```python
from build123d import *

# Parameters (mm, degrees)
F0_W     = 40
F0_H     = 20
F1_DEPTH = 700
F2_SIZE2 = 3.52653
F2_SIZE  = 19.99999
F3_SIZE2 = 3.52653
F3_SIZE  = 19.99999


# Not quite as in the source:
# - a fillet or chamfer is up to 0.001 mm smaller than in the source, because OpenCascade refuses the exact size


with BuildPart() as f1:
    # F0 (on Front) → F1 (new body)
    with BuildSketch(Plane.XZ):
        with Locations((20, 10)):
            Rectangle(F0_W, F0_H)
    extrude(amount=F1_DEPTH)

    # F2 (size 20 and 3.5265396142 in the source; OpenCascade refuses exactly that, so slightly less here)
    f2_edges = [f1.edges().sort_by_distance(p)[0] for p in [
        (20, -700, 0),
    ]]
    f2_side = f1.faces().sort_by_distance((20, -700, 10))[0]
    chamfer(f2_edges, length=F2_SIZE, length2=F2_SIZE2, reference=f2_side)

    # F3 (size 20 and 3.5265396142 in the source; OpenCascade refuses exactly that, so slightly less here)
    f3_edges = [f1.edges().sort_by_distance(p)[0] for p in [
        (20, 0, 0),
    ]]
    f3_side = f1.faces().sort_by_distance((20, 0, 10))[0]
    chamfer(f3_edges, length=F3_SIZE, length2=F3_SIZE2, reference=f3_side)


solid = f1.part
```
Here's how the part is built. I have some questions about the finished solid (model axes, mm). Give positions to 0.01 mm unless a question says otherwise; leave off trailing zeros. Use a Markdown table: item, result. Add a question column.
1. For pin 1 Ø5 at (x, z) = (5, 9.5) entering from -Y; pin 2 Ø6 at (x, z) = (12.5, 3.5) entering from -Y; pin 3 Ø6 at (y, z) = (-169, 17) entering from -X; pin 4 Ø5 at (x, z) = (31, 15) entering from +Y, each with a flat end and sliding along its axis, tell me the tip position at first contact or that it passes through.
2. I need wall thicknesses on probe 1 along Y at (x, z) = (29.5, 10.75); probe 2 along Y at (x, z) = (4.5, 1.5). Which ranges of each line are inside material? Lowest first, please. Write a range as from..to.
3. If we mould it in two halves opening along Y, with no side actions, what happens to faces 1 (the flat face through (40, -345, 10)), 2 (the flat face through (19.72, -698.212, 9.86)), 3 (the flat face through (19.72, -1.788, 9.86))? For each: +Y half, -Y half, draft (parallel to the pull), parting line (faces both ways), or undercut.
Results list:
| question | item | result |
|---|---|---|
| 1 | pin 1 | stops at y = -698.59 |
| 1 | pin 2 | stops at y = -697.62 |
| 1 | pin 3 | stops at x = 0 |
| 1 | pin 4 | stops at y = -0.44 |
| 2 | probe 1 | y = -698.37..-1.63 |
| 2 | probe 2 | y = -696.74..-3.26 |
| 3 | face 1 | draft |
| 3 | face 2 | -Y half |
| 3 | face 3 | +Y half |
